Read the model definition and answer for the solid it produces. Units are mm, in the model's axes. Coordinates: 2 decimals unless noted, no trailing zeros. Write each loop counter-clockwise with the first axis right and the second up, starting at its lowest first coordinate (ties: lowest second). Pieces come first, ordered by that corner, then holes. Notation, with made-up numbers: (86.25, -21) -> (96.25, -21) arc R38 ccw to (96.25, 17) -> close; hole circle Ø10 at (-38.75, -35). An arc over 180 degrees is marked (long way). Answer in a Markdown table with one row per item. Add a question column.
Item 1: Section C-C on z = 1.6 is taken. Write down the section's boundary in (x, y), then the cut area to 3 significant figures.
Item 2: Straight lines are drawn through the part: line 1 (Y direction, x = -8, z = 0.8); line 2 (X direction, y = 8, z = 0.6); line 3 (Y direction, x = 39, z = 1). For each, find the intervals that lie inside material, in ascending order. Write a range as from..to.
Item 3: Given pin 1 Ø5 at (x, y) = (-8, 55) entering from +Z, flat-ended and moving along its own axis, determine where the tip first touches the part or whether it passes through.
Item 4: Section D-D on y = 55 is taken. Write down the section's boundary in (x, z), then the cut area to 4 significant figures.
Item 5: Section B-B on x = 20 is taken. Write down the section's boundary in (y, z).
Item 6: Section A-A on y = 8 is taken. Write down the section's boundary in (x, z), then the cut area to 3 significant figures.
Autodesk Inventor part; units mm, degrees
ref_plane "YZ Plane" through (0, 0, 0) normal (1, 0, 0) x (0, 1, 0)
ref_plane "XZ Plane" through (0, 0, 0) normal (0, 1, 0) x (-1, 0, 0)
ref_plane "XY Plane" through (0, 0, 0) normal (0, 0, 1) x (1, 0, 0)
sketch "草图1" plane through (0, 0, 0) normal (0, 0, 1) x (1, 0, 0)
  line L0 (0, 0) -> (-16, 0)
  line L1 (-16, 0) -> (-16, 65)
  line L2 (-16, 65) -> (0, 65)
  line L3 (0, 65) -> (0, 0)
  line L4 (-16, 16) -> (49, 16)
  line L5 (49, 16) -> (49, 0)
  line L6 (49, 0) -> (-16, 0)
  line L7 (-16, 0) -> (-16, 16)
  line L8 (-8, 65) -> (-8, 0)
  line L9 (-16, 8) -> (49, 8)
  circle A0 centre (-8, 55) radius 2.75
  circle A1 centre (-8, 36) radius 2.75
  circle A2 centre (39, 8) radius 2.75
  circle A3 centre (20, 8) radius 2.75
  point P0 (0, 16)
  dimension "d0" = 65
  dimension "d1" = 65
  dimension "d2" = 16
  dimension "d3" = 16
  dimension "d4" = 5.5
  dimension "d5" = 5.5
  dimension "d6" = 19
  dimension "d7" = 10
  dimension "d8" = 5.5
  dimension "d9" = 5.5
  dimension "d10" = 19
  dimension "d11" = 10
extrude "拉伸1" add sketch "草图1" along normal blind 2.5 contours L0 L8 L9 L3 | L3 L9 A3 A2 L5 L6 | L0 L1 L9 L8 | L9 L8 L4 L3 | L3 L4 L5 L9 A2 A3 | L9 L1 L4 L8 | L4 L8 A1 A0 L2 L3 | L4 L1 L2 L8 A0 A1
properties part number "L型"
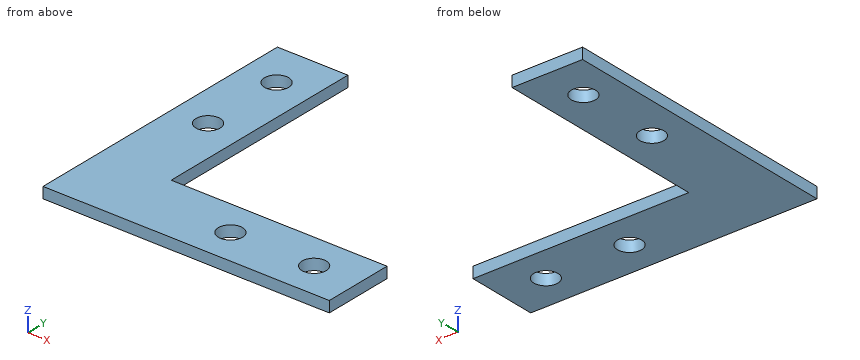
Results below:
| question | item | result |
|---|---|---|
| 1 | outline | (-16, 0) -> (49, 0) -> (49, 16) -> (0, 16) -> (0, 65) -> (-16, 65) -> close; hole circle Ø5.5 at (-8, 36); hole circle Ø5.5 at (-8, 55); hole circle Ø5.5 at (20, 8); hole circle Ø5.5 at (39, 8) |
| 1 | area | 1,730 mm2 |
| 2 | line 1 | y = 0..33.25, 38.75..52.25, 57.75..65 |
| 2 | line 2 | x = -16..17.25, 22.75..36.25, 41.75..49 |
| 2 | line 3 | y = 0..5.25, 10.75..16 |
| 3 | pin 1 | passes through |
| 4 | outline | (-16, 0) -> (-10.75, 0) -> (-10.75, 2.5) -> (-16, 2.5) -> close; (-5.25, 0) -> (0, 0) -> (0, 2.5) -> (-5.25, 2.5) -> close |
| 4 | area | 26.25 mm2 |
| 5 | outline | (0, 0) -> (5.25, 0) -> (5.25, 2.5) -> (0, 2.5) -> close; (10.75, 0) -> (16, 0) -> (16, 2.5) -> (10.75, 2.5) -> close |
| 6 | outline | (-16, 0) -> (17.25, 0) -> (17.25, 2.5) -> (-16, 2.5) -> close; (22.75, 0) -> (36.25, 0) -> (36.25, 2.5) -> (22.75, 2.5) -> close; (41.75, 0) -> (49, 0) -> (49, 2.5) -> (41.75, 2.5) -> close |
| 6 | area | 135 mm2 |
